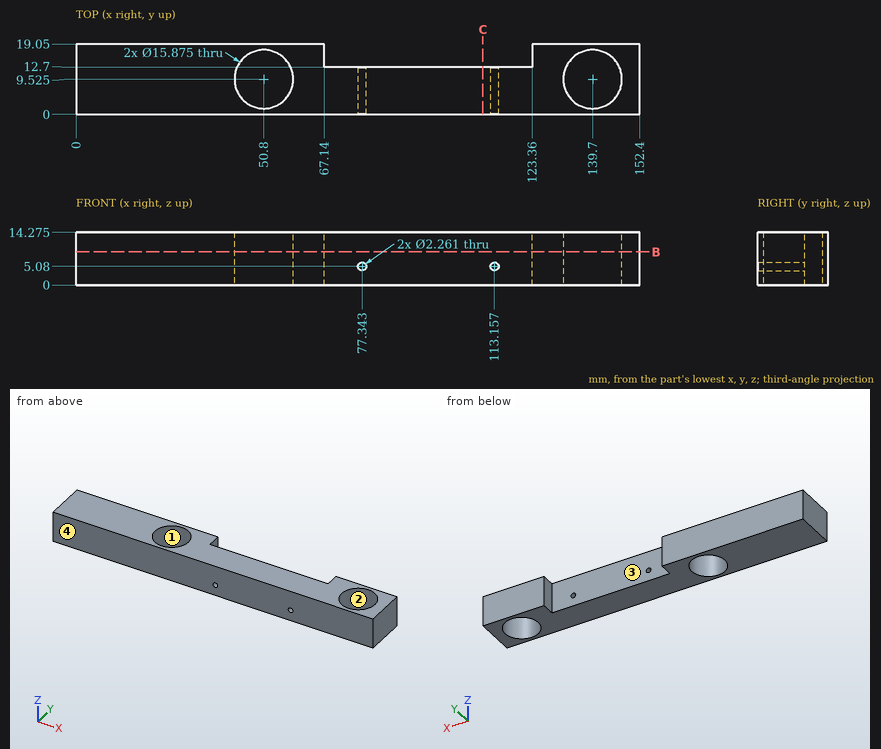
The figure shows three views and two pictorial views of one solid part (mm, origin at its lowest corner). Answer the questions. Round coordinates to 2 decimals unless told otherwise and drop trailing zeros. Loops run counter-clockwise (first coordinate to the right, second up) from the corner with the lowest first, then second, coordinate; pieces in that order, holes last. Notation, with made-up numbers: (-17.75, -23) - (35.25, -23) arc R29 cw to (35.25, 10) - close; hole circle Ø5 at (84, 46). An arc over 180 degrees is marked (long way). Use one line per item in the form item = value. Start each with the question number.
(1) Determine the mould class of the marked faces 1, 2, 3 and 4 for opening direction Y: +Y half, -Y half, draft (parallel to the pull), parting line (faces both ways), or undercut.
(2) Flat-ended cylindrical pins translate along their axes: P1, Ø5, axis at x = 94.5, z = 10, coming from the +Y side; P2, Ø1.4, axis at x = 77.343, z = 5.08, coming from the -Y side. Find the tip coordinate at first contact, or state that the pin passes through.
(3) Find section C-C on x = 110. Determine the outline of the cut face in (y, z) (1 decimal).
(4) Find section B-B on z = 9. Give the number of separate pieces and of enclosed holes in the cut face, and give its area (3 significant figures).
(5) Consider line 1 (X direction, y = 14, z = 13.25) (1 decimal); line 2 (X direction, y = 3.75, z = 8.25) (1 decimal); line 3 (X direction, y = 2.5, z = 13.5) (1 decimal). Determine where each line is inside the solid, lowest interval first.
Answer list:
q1.face_1 = undercut
q1.face_2 = undercut
q1.face_3 = +Y half
q1.face_4 = -Y half
q2.P1 = 12.7
q2.P2 = through
q3.outline = (0, 0) - (12.7, 0) - (12.7, 14.3) - (0, 14.3) - close
q4.separate_pieces = 1
q4.enclosed_holes = 2
q4.area = 2,150 mm^2
q5.line_1 = 0 to 44.2, 57.4 to 67.1, 123.4 to 133.1, 146.3 to 152.4
q5.line_2 = 0 to 45.4, 56.2 to 134.3, 145.1 to 152.4
q5.line_3 = 0 to 47.1, 54.5 to 136, 143.4 to 152.4
